from build123d import *

# Parameters (mm, degrees)
F0_W     = 12
F0_H     = 12
F0_R     = 2.9845
F1_DEPTH = 18
F2_R     = 1.75
F3_DEPTH = 25.4
F4_R     = 5.08


with BuildPart() as f1:
    # F0 (on Front) → F1 (new body)
    with BuildSketch(Plane.XZ):
        with Locations((-14.06993, 28.901128)):
            Rectangle(F0_W, F0_H)
        with Locations((-14.06993, 28.901128)):
            Circle(F0_R, mode=Mode.SUBTRACT)
        Polygon((-8.06993, 42.901128), (-8.06993, 34.901128), (-8.06993, 22.901128), (-3.49793, 22.901128), (-3.49793, 42.901128), align=None)
    extrude(amount=F1_DEPTH)

    # F2 (on face) → F3 (cut)
    with BuildSketch(Plane(origin=(-8.06993, 0, 0), x_dir=(0, -1, 0), z_dir=(-1, 0, 0))):
        with Locations((4, 38.901128)):
            Circle(F2_R)
        with Locations((14, 38.901128)):
            Circle(F2_R)
    extrude(amount=-F3_DEPTH, mode=Mode.SUBTRACT)

    # F4
    f4_edges = [f1.edges().sort_by_distance(p)[0] for p in [
        (-5.78393, 0, 42.901128),
        (-5.78393, -18, 42.901128),
        (-20.06993, -9, 34.901128),
        (-20.06993, -9, 22.901128),
        (-3.49793, -9, 22.901128),
    ]]
    fillet(f4_edges, radius=F4_R)


solid = f1.part
Work out the finished part from the listing and answer in its coordinate system (mm). A direction names the side the tool comes from. Give positions to 0.01 mm unless a question says otherwise; leave off trailing zeros. Write each loop counter-clockwise with the first axis right and the second up, starting at its lowest first coordinate (ties: lowest second). Pieces come first, ordered by that corner, then holes. Notation, with made-up numbers: M 25,49 L 56,49 A16 cw 56,80 Z; hole C 86,40 d6. An arc over 180 degrees is marked long. Answer as CSV lines item,"result".
Q1. A cutting plane is placed at A-A on y = -4. Write down the section's boundary in (x, z) (1 decimal).
A:
outline,"M -20.1,28 A5.1 ccw -15,22.9 L -8.6,22.9 A5.1 ccw -3.5,28 L -3.5,37.2 L -8.1,37.2 L -8.1,34.9 L -15,34.9 A5.1 ccw -20.1,29.8 Z; M -8.1,40.7 L -3.5,40.7 L -3.5,42.8 L -8.1,42.8 Z; hole C -14.1,28.9 d6"
Q2. A cutting plane is placed at D-D on y = -8. Write down the section's boundary in (x, z), plus the area to 3 significant figures.
A:
outline,"M -20.07,27.98 A5.08 ccw -14.99,22.9 L -8.58,22.9 A5.08 ccw -3.5,27.98 L -3.5,42.9 L -8.07,42.9 L -8.07,34.9 L -14.99,34.9 A5.08 ccw -20.07,29.82 Z; hole C -14.07,28.9 d5.97"
area,"191 mm²"
Q3. The mould has two halves that part along X. Classify faces 1 (the cylindrical face through (-11.313, -8.874, 27.758)), 2 (the cylindrical face through (-18.621, -9.126, 33.374)), 3 (the flat face through (-12, -9, 22.901)): +X half, -X half, draft (parallel to the pull), parting line (faces both ways), or undercut.
A:
face 1,"undercut"
face 2,"-X half"
face 3,"draft"
Q4. A cutting plane is placed at C-C on y = -14.75. Write down the section's boundary in (x, z).
A:
outline,"M -20.07,27.98 A5.08 ccw -14.99,22.9 L -8.58,22.9 A5.08 ccw -3.5,27.98 L -3.5,37.32 L -8.07,37.32 L -8.07,34.9 L -14.99,34.9 A5.08 ccw -20.07,29.82 Z; M -8.07,40.48 L -3.5,40.48 L -3.5,42.56 L -8.07,42.56 Z; hole C -14.07,28.9 d5.97"
Q5. A tool of negligible diameter and unlimited length cuts with its end or side. For faces 4 (the flat face through (-10, -18, 29)), 5 (the flat face through (-12, -9, 34.901)), from which of +Z, -Z, +X, -X, +Y, -Y can it reach the whole face along a straight path? Write none if from no direction.
A:
face 4,"+Z, -Z, +X, -X, -Y"
face 5,"+Z, -X, +Y, -Y"
Q6. Find the intervals of material crossed by probe 1 along X at (y, z) = (-8.25, 40.75); probe 2 along Z at (x, y) = (-5.5, -4) (3 decimals); probe 3 along Z at (x, y) = (-7.25, -3), in increasing order. Write a range as [from, to].
A:
probe 1,"x = [-8.07, -3.5]"
probe 2,"z = [23.94, 37.151], [40.651, 42.785]"
probe 3,"z = [23.08, 37.46], [40.34, 42.46]"
Q7. A cutting plane is placed at B-B on x = -12.5. Write down the section's boundary in (y, z).
A:
outline,"M -18,22.9 L 0,22.9 L 0,26.36 L -18,26.36 Z; M -18,31.44 L 0,31.44 L 0,34.9 L -18,34.9 Z"
Q8. Given P1, Ø6, axis at x = -18, y = -3.5, coming from the +Z side; P2, Ø3.5, axis at x = -14.07, z = 28.9, coming from the -Y side; P3, Ø4.5, axis at y = -4, z = 38.9, coming from the -X side; P4, Ø1, axis at x = -7, y = -10, coming from the -Z side, each flat-ended and moving along its own axis, determine where each tip first touches the part or whether it passes through.
A:
P1,"stops at z = 34.9"
P2,"passes through"
P3,"stops at x = -8.07"
P4,"stops at z = 23.02"
